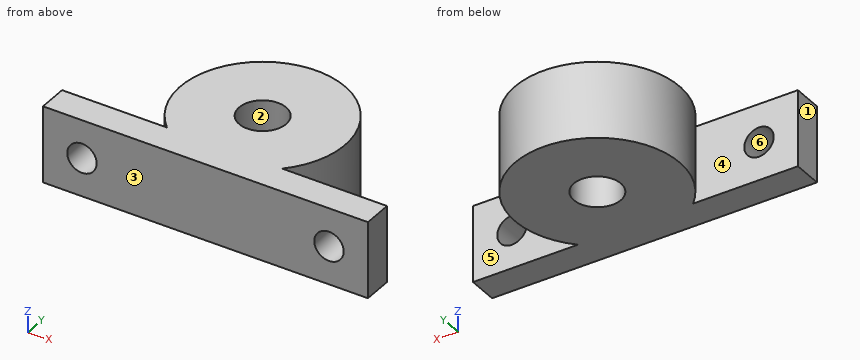
from build123d import *

# Parameters (mm, degrees)
SKETCH1_R           = 4
BOSS_EXTRUDE1_DEPTH = 13
SKETCH2_R           = 2.5
CUT_EXTRUDE1_DEPTH  = 30


with BuildPart() as part:
    # Sketch1 → Boss-Extrude1 (new body)
    with BuildSketch(Plane.XY):
        with BuildLine():
            Line((-27.625, -15), (27.625, -15))
            Line((27.625, -15), (27.625, -10))
            Line((27.625, -10), (9.797958971, -10))
            ThreePointArc((9.797958971, -10), (0, 14), (-9.797958971, -10))
            Line((-9.797958971, -10), (-27.625, -10))
            Line((-27.625, -10), (-27.625, -15))
        make_face()
        Circle(SKETCH1_R, mode=Mode.SUBTRACT)
    extrude(amount=BOSS_EXTRUDE1_DEPTH)

    # Sketch2 → Cut-Extrude1 (cut, through all)
    with BuildSketch(Plane.XZ.offset(15)):
        with Locations((-21, 6.5)):
            Circle(SKETCH2_R)
        with Locations((21, 6.5)):
            Circle(SKETCH2_R)
    extrude(amount=-CUT_EXTRUDE1_DEPTH, mode=Mode.SUBTRACT)


solid = part.part
Verification items for the finished model (mm, model axes). Face numbers are marked on the shaded views. A direction names the side the tool comes from. Coordinates: 2 decimals unless noted, no trailing zeros. Order: outer loops, then holes, each group sorted by start corner. A loop starts at its lowest first (then second) coordinate and runs counter-clockwise, first axis right, second up. Notation, with made-up numbers: (-12.75, 42) -> (-1.75, 42) arc R12 cw to (-1.75, 64) -> close; hole circle Ø8 at (-3, -33). An arc over 180 degrees is marked (long way). Put each result on its own line as item: value. Start each with the question number.
1. Cross-section at D-D, the plane z = 2.5. Record the boundary of the cut face in (x, y) (3 decimals), then the cut area to 3 significant figures.
2. Cross-section at C-C, the plane z = 6.5. Record the boundary of the cut face in (x, y) (3 decimals).
3. Cross-section at B-B, the plane x = 0. Record the boundary of the cut face in (y, z), then the cut area to 3 significant figures.
4. Cross-section at A-A, the plane y = 0. Record the boundary of the cut face in (x, z).
5. Material ranges on L1, parallel to Z at x = 21, y = -12.55; L2, parallel to Y at x = -13, z = 7.75; L3, parallel to X at y = -0.75, z = 2, recorded low to high. Write a range as [from, to].
6. Access from +Z, -Z, +X, -X, +Y, -Y to the whole of each face (thin tool, end or side, straight path). Record for the marked faces 5 and 6.
7. Go/stop test with flat-tipped pins: pin 1 Ø5 at (x, y) = (7.5, 7.5) entering from -Z; pin 2 Ø6.5 at (x, y) = (0, 0) entering from +Z; pin 3 Ø4 at (y, z) = (9, 8) entering from +X; pin 4 Ø3 at (y, z) = (4.5, 10) entering from -X. Record where each tip stops, or that it passes through.
8. Mould release check, pull along Y, two halves, no side actions. Record for the marked faces 1, 2, 3 and 4: released by +Y, released by -Y, zero draft, split by the parting line, or undercut.
Computed:
1. outline: (-27.625, -15) -> (27.625, -15) -> (27.625, -10) -> (9.798, -10) arc R14 ccw (long way) to (-9.798, -10) -> (-27.625, -10) -> close; hole circle Ø8 at (0, 0)
1. area: 788 mm2
2. outline: (-27.625, -15) -> (-23.5, -15) -> (-23.5, -10) -> (-27.625, -10) -> close; (-18.5, -15) -> (18.5, -15) -> (18.5, -10) -> (9.798, -10) arc R14 ccw (long way) to (-9.798, -10) -> (-18.5, -10) -> close; (23.5, -15) -> (27.625, -15) -> (27.625, -10) -> (23.5, -10) -> close; hole circle Ø8 at (0, 0)
3. outline: (-15, 0) -> (-4, 0) -> (-4, 13) -> (-15, 13) -> close; (4, 0) -> (14, 0) -> (14, 13) -> (4, 13) -> close
3. area: 273 mm2
4. outline: (-14, 0) -> (-4, 0) -> (-4, 13) -> (-14, 13) -> close; (4, 0) -> (14, 0) -> (14, 13) -> (4, 13) -> close
5. L1: [0, 4], [9, 13]
5. L2: [-15, -10], [-5.2, 5.2]
5. L3: [-13.98, -3.93], [3.93, 13.98]
6. face 5: +Z, -Z, +X
6. face 6: +Y, -Y
7. pin 1: z = 0
7. pin 2: through
7. pin 3: x = 12.12
7. pin 4: x = -13.67
8. face 1: zero draft
8. face 2: undercut
8. face 3: released by -Y
8. face 4: undercut
